Verification items for the finished model (mm, model axes). A direction names the side the tool comes from. Round coordinates to 2 decimals unless told otherwise and drop trailing zeros. Loops run counter-clockwise (first coordinate to the right, second up) from the corner with the lowest first, then second, coordinate; pieces in that order, holes last. Notation, with made-up numbers: M -40,-35 L -18,-35 A12 ccw -18,-25 Z; hole C 28,34 d9. An arc over 180 degrees is marked long. One line per item, written item: value.
from build123d import *

# Parameters (mm, degrees)
SKETCH1_R           = 240
BOSS_EXTRUDE1_DEPTH = 700
SKETCH2_R           = 230
CUT_EXTRUDE1_DEPTH  = 10
CUT_EXTRUDE2_START  = -10
SKETCH3_R           = 230
CUT_EXTRUDE2_DEPTH  = 10
CUT_EXTRUDE3_REACH  = 770.96
SKETCH5_R           = 16.25
BOSS_EXTRUDE2_DEPTH = 150
BOSS_EXTRUDE3_START = 150
SKETCH6_R           = 16.25
BOSS_EXTRUDE3_DEPTH = 150
SKETCH7_R           = 12
CUT_EXTRUDE4_DEPTH  = 50
CUT_EXTRUDE5_START  = -50
SKETCH8_R           = 12
CUT_EXTRUDE5_DEPTH  = 50
CUT_EXTRUDE8_START  = -45
CUT_EXTRUDE8_DEPTH  = 45


with BuildPart() as part:
    # Sketch1 → Boss-Extrude1 (new body)
    with BuildSketch(Plane.XY):
        Circle(SKETCH1_R)
    extrude(amount=BOSS_EXTRUDE1_DEPTH)

    # Sketch2 → Cut-Extrude1 (cut)
    with BuildSketch(Plane.XY.offset(700)):
        Circle(SKETCH2_R)
    extrude(amount=-CUT_EXTRUDE1_DEPTH, mode=Mode.SUBTRACT)

    # Sketch3 → Cut-Extrude2 (cut)
    with BuildSketch(Plane(origin=(0, 0, 0), x_dir=(-1, 0, 0), z_dir=(0, 0, -1)).offset(CUT_EXTRUDE2_START)):
        with Locations(Location((0, 0, 0), (0, 0, 180))):
            Circle(SKETCH3_R)
    extrude(amount=CUT_EXTRUDE2_DEPTH, mode=Mode.SUBTRACT)

    # Sketch4 → Cut-Extrude3 (cut, up to next)
    with BuildSketch(Plane.XY.offset(690), mode=Mode.PRIVATE) as cut_extrude3_sk1:
        with BuildLine():
            Line((-5.578158138, 213.912523134), (-14.650908758, 40.79412842))
            ThreePointArc((-14.650908758, 40.79412842), (-15.620272478, 37.825559391), (-17.95016171, 35.746212311))
            ThreePointArc((-17.95016171, 35.746212311), (-28.284271247, 28.284271247), (-35.746212311, 17.95016171))
            ThreePointArc((-35.746212311, 17.95016171), (-37.825559391, 15.620272478), (-40.79412842, 14.650908758))
            Line((-40.79412842, 14.650908758), (-213.912523134, 5.578158138))
            ThreePointArc((-213.912523134, 5.578158138), (-221.577643537, 8.564792629), (-224.409644682, 16.288381554))
            ThreePointArc((-224.409644682, 16.288381554), (-159.099025767, 159.099025767), (-16.288381554, 224.409644682))
            ThreePointArc((-16.288381554, 224.409644682), (-8.564792629, 221.577643537), (-5.578158138, 213.912523134))
        make_face()
    cut_extrude3_tool1 = extrude(cut_extrude3_sk1.sketch, amount=-CUT_EXTRUDE3_REACH, mode=Mode.PRIVATE) & part.part
    # Sketch4 → Cut-Extrude3 (cut, up to next)
    with BuildSketch(Plane.XY.offset(690), mode=Mode.PRIVATE) as cut_extrude3_sk2:
        with BuildLine():
            Line((5.578158138, 213.912523134), (14.650908758, 40.79412842))
            ThreePointArc((14.650908758, 40.79412842), (15.620272478, 37.825559391), (17.95016171, 35.746212311))
            ThreePointArc((17.95016171, 35.746212311), (28.284271247, 28.284271247), (35.746212311, 17.95016171))
            ThreePointArc((35.746212311, 17.95016171), (37.825559391, 15.620272478), (40.79412842, 14.650908758))
            Line((40.79412842, 14.650908758), (213.912523134, 5.578158138))
            ThreePointArc((213.912523134, 5.578158138), (221.577643537, 8.564792629), (224.409644682, 16.288381554))
            ThreePointArc((224.409644682, 16.288381554), (159.099025767, 159.099025767), (16.288381554, 224.409644682))
            ThreePointArc((16.288381554, 224.409644682), (8.564792629, 221.577643537), (5.578158138, 213.912523134))
        make_face()
    cut_extrude3_tool2 = extrude(cut_extrude3_sk2.sketch, amount=-CUT_EXTRUDE3_REACH, mode=Mode.PRIVATE) & part.part
    # Sketch4 → Cut-Extrude3 (cut, up to next)
    with BuildSketch(Plane.XY.offset(690), mode=Mode.PRIVATE) as cut_extrude3_sk3:
        with BuildLine():
            Line((-213.912523134, -5.578158138), (-40.79412842, -14.650908758))
            ThreePointArc((-40.79412842, -14.650908758), (-37.825559391, -15.620272478), (-35.746212311, -17.95016171))
            ThreePointArc((-35.746212311, -17.95016171), (-28.284271247, -28.284271247), (-17.95016171, -35.746212311))
            ThreePointArc((-17.95016171, -35.746212311), (-15.620272478, -37.825559391), (-14.650908758, -40.79412842))
            Line((-14.650908758, -40.79412842), (-5.578158138, -213.912523134))
            ThreePointArc((-5.578158138, -213.912523134), (-8.564792629, -221.577643537), (-16.288381554, -224.409644682))
            ThreePointArc((-16.288381554, -224.409644682), (-159.099025767, -159.099025767), (-224.409644682, -16.288381554))
            ThreePointArc((-224.409644682, -16.288381554), (-221.577643537, -8.564792629), (-213.912523134, -5.578158138))
        make_face()
    cut_extrude3_tool3 = extrude(cut_extrude3_sk3.sketch, amount=-CUT_EXTRUDE3_REACH, mode=Mode.PRIVATE) & part.part
    # Sketch4 → Cut-Extrude3 (cut, up to next)
    with BuildSketch(Plane.XY.offset(690), mode=Mode.PRIVATE) as cut_extrude3_sk4:
        with BuildLine():
            Line((213.912523134, -5.578158138), (40.79412842, -14.650908758))
            ThreePointArc((40.79412842, -14.650908758), (37.825559391, -15.620272478), (35.746212311, -17.95016171))
            ThreePointArc((35.746212311, -17.95016171), (28.284271247, -28.284271247), (17.95016171, -35.746212311))
            ThreePointArc((17.95016171, -35.746212311), (15.620272478, -37.825559391), (14.650908758, -40.79412842))
            Line((14.650908758, -40.79412842), (5.578158138, -213.912523134))
            ThreePointArc((5.578158138, -213.912523134), (8.564792629, -221.577643537), (16.288381554, -224.409644682))
            ThreePointArc((16.288381554, -224.409644682), (159.099025767, -159.099025767), (224.409644682, -16.288381554))
            ThreePointArc((224.409644682, -16.288381554), (221.577643537, -8.564792629), (213.912523134, -5.578158138))
        make_face()
    cut_extrude3_tool4 = extrude(cut_extrude3_sk4.sketch, amount=-CUT_EXTRUDE3_REACH, mode=Mode.PRIVATE) & part.part
    add(cut_extrude3_tool1.solids().sort_by_distance((-101.943067, 101.943067, 690))[0], mode=Mode.SUBTRACT)
    add(cut_extrude3_tool2.solids().sort_by_distance((101.943067, 101.943067, 690))[0], mode=Mode.SUBTRACT)
    add(cut_extrude3_tool3.solids().sort_by_distance((-101.943067, -101.943067, 690))[0], mode=Mode.SUBTRACT)
    add(cut_extrude3_tool4.solids().sort_by_distance((101.943067, -101.943067, 690))[0], mode=Mode.SUBTRACT)

    # Sketch5 → Boss-Extrude2 (add)
    with BuildSketch(Plane.XY.offset(690)):
        Circle(SKETCH5_R)
    extrude(amount=BOSS_EXTRUDE2_DEPTH)

    # Sketch6 → Boss-Extrude3 (add)
    with BuildSketch(Plane(origin=(0, 0, 10), x_dir=(-1, 0, 0), z_dir=(0, 0, -1)).offset(BOSS_EXTRUDE3_START)):
        with Locations(Location((0, 0, 0), (0, 0, 180))):
            Circle(SKETCH6_R)
    extrude(amount=-BOSS_EXTRUDE3_DEPTH)

    # Sketch7 → Cut-Extrude4 (cut)
    with BuildSketch(Plane.XY.offset(840)):
        Circle(SKETCH7_R)
    extrude(amount=-CUT_EXTRUDE4_DEPTH, mode=Mode.SUBTRACT)

    # Sketch8 → Cut-Extrude5 (cut)
    with BuildSketch(Plane(origin=(0, 0, -140), x_dir=(-1, 0, 0), z_dir=(0, 0, -1)).offset(CUT_EXTRUDE5_START)):
        with Locations(Location((0, 0, 0), (0, 0, 180))):
            Circle(SKETCH8_R)
    extrude(amount=CUT_EXTRUDE5_DEPTH, mode=Mode.SUBTRACT)

    # Sketch10 → Cut-Extrude8 (cut)
    with BuildSketch(Plane(origin=(0, 0, -140), x_dir=(-1, 0, 0), z_dir=(0, 0, -1)).offset(CUT_EXTRUDE8_START)):
        with BuildLine():
            Line((-4, 11.313708499), (-4, 15.003708499))
            Line((-4, 15.003708499), (4, 15.003708499))
            Line((4, 15.003708499), (4, 11.313708499))
            ThreePointArc((4, 11.313708499), (0, 12), (-4, 11.313708499))
        make_face()
    extrude(amount=CUT_EXTRUDE8_DEPTH, mode=Mode.SUBTRACT)


solid = part.part
(1) Thickness scan on L1, parallel to Y at x = 0, z = 825; L2, parallel to X at y = -43.5, z = 438; L3, parallel to X at y = -167, z = 619.5. Record the ranges inside material, lowest first. Write a range as from..to.
Completed:
L1: y = -16.25..-12, 12..16.25
L2: x = -236.02..-220.75, -14.51..14.51, 220.75..236.02
L3: x = -172.37..-150.78, -8.04..8.04, 150.78..172.37
(2) Depth check by flat-ended pin: pin 1 Ø21.5 at (x, y) = (0, 0) entering from -Z; pin 2 Ø3 at (y, z) = (12.5, -115) entering from -X; pin 3 Ø5 at (y, z) = (-41.5, 698) entering from -X. Enter the tip coordinate at first touch or a pass-through.
Completed:
pin 1: stops at z = -90
pin 2: stops at x = -11.96
pin 3: stops at x = -236.81
(3) Sectioned sample at B-B on y = 161.5. Enter the section's corners in (x, z).
Completed:
outline: M -177.53,0 L -163.76,0 L -163.76,10 L -156.66,10 L -156.66,690 L -163.76,690 L -163.76,700 L -177.53,700 Z; M -8.32,10 L 8.32,10 L 8.32,690 L -8.32,690 Z; M 156.66,10 L 163.76,10 L 163.76,0 L 177.53,0 L 177.53,700 L 163.76,700 L 163.76,690 L 156.66,690 Z
(4) Sectioned sample at A-A on z = 190.5. Count the separate pieces of the cut face and the enclosed holes in it, and give its area (3 significant figures).
Completed:
separate pieces: 1
enclosed holes: 4
area: 41,900 mm^2
(5) Tool access check on faces 5 (the face through (-10.18, -126.14, 354.76)), 6 (the face through (15.5, 4.88, 763.95)), 7 (the face through (16, 16, 10)). Record the directions out of +Z, -Z, +X, -X, +Y, -Y that give a thin tool (end or side, any length) a straight path to the whole face; none if there is none.
Completed:
face 5: +Z, -Z
face 6: +Z
face 7: -Z
(6) Sectioned sample at C-C on x = 103.5. Enter the section's corners in (y, z).
Completed:
outline: M -216.54,0 L -205.4,0 L -205.4,10 L -199.78,10 L -199.78,690 L -205.4,690 L -205.4,700 L -216.54,700 Z; M -11.36,10 L 11.36,10 L 11.36,690 L -11.36,690 Z; M 199.78,10 L 205.4,10 L 205.4,0 L 216.54,0 L 216.54,700 L 205.4,700 L 205.4,690 L 199.78,690 Z
(7) Mould release check, pull along Y, two halves, no side actions. Record for faces 1 (the face through (-239.77, 10.55, 345.1)), 2 (the face through (1.13, -12.11, -140)), 3 (the face through (-160.68, 157.5, 354.76)), 4 (the face through (16, -16, 690)): +Y half, -Y half, draft (parallel to the pull), parting line (faces both ways), or undercut.
Completed:
face 1: parting line
face 2: draft
face 3: undercut
face 4: undercut
